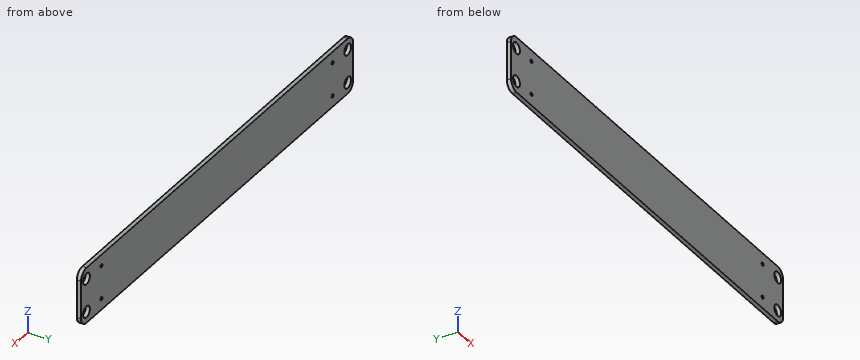
from build123d import *

# Parameters (mm, degrees)
SKETCH1_R           = 6.35
SKETCH1_R_2         = 1.905
BOSS_EXTRUDE1_DEPTH = 4.7625


with BuildPart() as part:
    # Sketch1 → Boss-Extrude1 (new body)
    with BuildSketch(Plane(origin=(0, 0, 0), x_dir=(1, 0, 0), z_dir=(0, 1, 0))):
        with BuildLine():
            Line((10.16, 0), (253.0475, 0))
            Line((253.0475, 0), (253.0475, -63.5))
            Line((253.0475, -63.5), (10.16, -63.5))
            ThreePointArc((10.16, -63.5), (2.975795103, -60.524204897), (0, -53.34))
            Line((0, -53.34), (0, -43.815))
            Line((0, -43.815), (0, -26.035))
            Line((0, -26.035), (0, -10.16))
            ThreePointArc((0, -10.16), (2.975795103, -2.975795103), (10.16, 0))
        make_face()
        with Locations((10.16, -50.8)):
            Circle(SKETCH1_R, mode=Mode.SUBTRACT)
        with Locations((10.16, -12.7)):
            Circle(SKETCH1_R, mode=Mode.SUBTRACT)
        with Locations((38.1, -50.8)):
            Circle(SKETCH1_R_2, mode=Mode.SUBTRACT)
        with Locations((38.1, -12.7)):
            Circle(SKETCH1_R_2, mode=Mode.SUBTRACT)
    boss_extrude1 = extrude(amount=BOSS_EXTRUDE1_DEPTH)

    # Mirror1: Boss-Extrude1 across plane
    add(boss_extrude1.mirror(Plane(origin=(253.0475, 4.7625, 0), x_dir=(0, 0, 1), z_dir=(-1, 0, 0))))


solid = part.part
Can you work these out from the model? Positions are in its coordinate system, mm. Round coordinates to 2 decimals unless told otherwise and drop trailing zeros. Use a Markdown table: item, result.
1) If I drill on line 1 along X through (y, z) = (2.9, 12.7) (3 decimals); line 2 along Z through (x, y) = (10.16, 3.1); line 3 along Z through (x, y) = (38, 0.35), over which ranges is the centre line in solid material (lowest first)?
Geometry says:
| item | result |
|---|---|
| line 1 | x = 0 to 3.81, 16.51 to 36.195, 40.005 to 466.09, 469.9 to 489.585, 502.285 to 506.095 |
| line 2 | z = 0 to 6.35, 19.05 to 44.45, 57.15 to 63.5 |
| line 3 | z = 0 to 10.8, 14.6 to 48.9, 52.7 to 63.5 |
2) Imagine slicing it at A-A (y = 3.6). Give the number of separate pieces and of enclosed holes in the cut face, then the cut area to 3 significant figures.
Geometry says:
| item | result |
|---|---|
| separate pieces | 1 |
| enclosed holes | 8 |
| area | 31,500 mm² |
3) I'm going to push a flat-ended pin straight in: P1, Ø10, axis at x = 10.16, z = 12.7, coming from the +Y side. Where does the tip first touch, or does it pass through?
Geometry says:
| item | result |
|---|---|
| P1 | passes through |
